Autodesk Inventor part; units mm, degrees
ref_plane "YZ Plane" through (0, 0, 0) normal (1, 0, 0) x (0, 1, 0)
ref_plane "XZ Plane" through (0, 0, 0) normal (0, 1, 0) x (-1, 0, 0)
ref_plane "XY Plane" through (0, 0, 0) normal (0, 0, 1) x (1, 0, 0)
sketch "スケッチ1" plane through (0, 0, 0) normal (0, 0, 1) x (1, 0, 0)
  line L0 (-5, 0) -> (0, 0)
  line L1 (-5, 0) -> (-5, -10)
  line L2 (0, -10) -> (-5, -10)
  line L3 (0, 0) -> (0, -10)
  line L4 (3.5355, 10.6066) -> (7.0711, 7.0711)
  line L5 (3.5355, 10.6066) -> (-3.5355, 3.5355)
  line L6 (0, 0) -> (-3.5355, 3.5355)
  line L7 (7.0711, 7.0711) -> (0, 0)
  line L8 (81.6459, 88.717) -> (85.1814, 85.1814)
  line L9 (81.6459, 88.717) -> (74.5748, 81.6459)
  line L10 (78.1104, 78.1104) -> (74.5748, 81.6459)
  line L11 (85.1814, 85.1814) -> (78.1104, 78.1104)
  line L12 (-5, -110.4647) -> (0, -110.4647)
  line L13 (-5, -110.4647) -> (-5, -120.4647)
  line L14 (0, -120.4647) -> (-5, -120.4647)
  line L15 (0, -110.4647) -> (0, -120.4647)
  line L16 (-4.4431, -120.4647) -> (-4.4431, 1.8404)
  line L17 (82.0397, 88.3232) -> (-4.4431, 1.8404)
  line L18 (60.4198, 56.1771) -> (5.0711, 0.8284)
  line L19 (5.0711, 0.8284) -> (23.6471, -6.866)
  arc A0 (60.4198, 56.1771) -> (23.6471, -6.866) centre (290.8276, -120.4647) ccw
  line L20 (94.3738, 75.989) -> (87.3027, 83.0601)
  arc A1 (87.3027, 83.0601) -> (3, -120.4647) centre (290.8276, -120.4647) ccw
  line L21 (13, -120.4647) -> (3, -120.4647)
  arc A2 (13.4052, -105.4647) -> (13, -120.4647) centre (290.8276, -120.4647) ccw
  arc A3 (94.3738, 75.989) -> (13.4052, -105.4647) centre (290.8276, -120.4647) ccw
  line L22 (85.1814, 85.1814) -> (0, 0)
  line L23 (0, 0) -> (0, -120.4647)
  line L24 (0, -120.4647) -> (3, -120.4647)
  arc A4 (87.3027, 83.0601) -> (3, -120.4647) centre (290.8276, -120.4647) ccw
  line L25 (87.3027, 83.0601) -> (85.1814, 85.1814)
  line L26 (3, -4.1716) -> (21.576, -11.866)
  arc A5 (21.576, -11.866) -> (3, -82.4465) centre (290.8276, -120.4647) ccw
  line L27 (3, -82.4465) -> (3, -4.1716)
  arc A6 (60.4198, 56.1771) -> (23.6471, -6.866) centre (290.8276, -120.4647) ccw
  line L28 (23.6471, -6.866) -> (5.0711, 0.8284)
  line L29 (5.0711, 0.8284) -> (60.4198, 56.1771)
  point P0 (74.9686, 81.2521)
  point P1 (3.9293, 10.2128)
  point P2 (-4.4431, -10)
  point P3 (-4.4431, -110.4647)
  point P4 (-3.1417, 3.1417)
  point P5 (-4.4431, 0)
  point P6 (0, -120.4647)
extrude "押し出し1" add sketch "スケッチ1" against normal blind 2.5 contours L7 L22 L11 L25 A1 L24 L15 L23 L3 | L2 L23 L12 L16 | L4 L17 L10 L22 | A1 L20 A3 A2 L21 | A0 L19 L18 | L26 A5 L27
sketch "スケッチ2" plane through (0, 0, 0) normal (0, 0, 1) x (1, 0, 0)
  circle A0 centre (8.0869, -115.4647) radius 1.5
  circle A1 centre (87.3027, 75.9801) radius 1.5
  point P0 (0, 0)
extrude "押し出し2" cut sketch "スケッチ2" against normal blind 10
properties part number "Spcer_curve" material "木材 (カエデ材)"
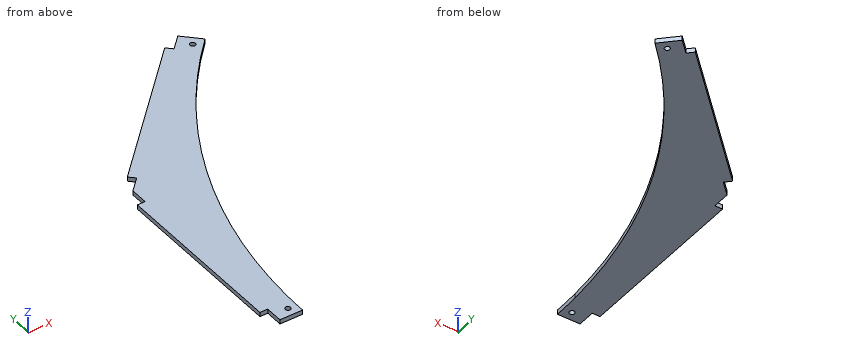
Could you check a few things on this model? Use its own coordinates, in mm. Give positions to 0.01 mm unless a question says otherwise; leave off trailing zeros. Loops run counter-clockwise (first coordinate to the right, second up) from the corner with the lowest first, then second, coordinate; pieces in that order, holes last. Notation, with made-up numbers: (56.25, 52) -> (60.25, 52) arc R24 cw to (60.25, 66) -> close; hole circle Ø3 at (68.25, -38.75). An arc over 180 degrees is marked (long way). Put each result on its own line as item: value.
(1) I'm going to push a flat-ended pin straight in: pin 1 Ø1.5 at (y, z) = (56.5, -1) entering from +X. Where does the tip first touch, or does it pass through?
Computed:
pin 1: x = 77.27
(2) Imagine slicing it at C-C on x = 46. Write out the boundary of the cut face in (y, z).
Computed:
outline: (10.87, -2.5) -> (52.28, -2.5) -> (52.28, 0) -> (10.87, 0) -> close
(3) Imagine slicing it at A-A on z = -0.6. Write out the boundary of the cut face in (x, y).
Computed:
outline: (-4.44, -110.46) -> (0, -110.46) -> (0, -120.46) -> (13, -120.46) arc R277.8 cw to (13.41, -105.46) arc R277.83 cw to (94.37, 75.99) -> (85.18, 85.18) -> (78.11, 78.11) -> (74.97, 81.25) -> (3.93, 10.21) -> (7.07, 7.07) -> (0, 0) -> (0, -10) -> (-4.44, -10) -> close; hole circle Ø3 at (8.09, -115.46); hole circle Ø3 at (87.3, 75.98)
(4) Imagine slicing it at B-B on y = -20. Write out the boundary of the cut face in (x, z), plus the area to 3 significant figures.
Computed:
outline: (-4.44, -2.5) -> (31.8, -2.5) -> (31.8, 0) -> (-4.44, 0) -> close
area: 90.6 mm^2
(5) Please list where these lines run through material, in increasing order: probe 1 along X at (y, z) = (19.5, -0.9); probe 2 along Y at (x, z) = (47, -1.05); probe 3 along Y at (x, z) = (50.5, -1.7). Write a range as [from, to].
Computed:
probe 1: [13.22, 50.83]
probe 2: [12.71, 53.28]
probe 3: [18.93, 56.78]
